Autodesk Inventor part; units mm, degrees
ref_plane "YZ Plane" through (0, 0, 0) normal (1, 0, 0) x (0, 1, 0)
ref_plane "XZ Plane" through (0, 0, 0) normal (0, 1, 0) x (-1, 0, 0)
ref_plane "XY Plane" through (0, 0, 0) normal (0, 0, 1) x (1, 0, 0)
sketch "Эскиз1" plane through (0, 0, 0) normal (0, 0, 1) x (1, 0, 0)
  line L0 (0, 0) -> (0, 7.5)
  line L1 (0, 7.5) -> (3, 7.5)
  line L2 (3, 7.5) -> (3, 2.5)
  line L3 (3, 2.5) -> (53, 2.5)
  line L4 (53, 2.5) -> (73.5263, 8)
  line L5 (128.4, 8) -> (128.4, 0)
  line L6 (128.4, 0) -> (0, 0)
  line L7 (107.9, 8) -> (107.9, 19)
  line L8 (107.9, 19) -> (106.9, 19)
  line L9 (106.9, 19) -> (106.9, 8)
  line L10 (73.5263, 8) -> (106.9, 8)
  line L11 (107.9, 8) -> (128.4, 8)
  dimension "d0" = 5
  dimension "d1" = 15
  dimension "d2" = 3
  dimension "d3" = 128.4
  dimension "d4" = 15
  dimension "d6" = 50
  dimension "d12" = 1
  dimension "d13" = 16
  dimension "d14" = 21.5
  dimension "d15" = 38
revolve "Вращение1" add sketch "Эскиз1" angle 360 about axis through (128.4, 0, 0) along (-1, 0, 0)
sketch "Эскиз2" plane through (0, 0, 0) normal (0, 1, 0) x (-1, 0, 0)
  circle A0 centre (-120.4, 0) radius 3
  line L0 (-128.4, 8) -> (-128.4, -8)
  point P0 (0, 0)
  point P1 (-128.4, 0)
  dimension "d8" = 6
  dimension "d9" = 8
extrude "Выдавливание1" cut sketch "Эскиз2" along normal through all both and the other way through all
properties part number "JF_0837B_Linear solenoid Pull 15N 12v1A Planger" material "Сталь, нержавеющая, аустенитная"
Verification items for the finished model (mm, model axes). A direction names the side the tool comes from. Give positions to 0.01 mm unless a question says otherwise; leave off trailing zeros. Loops run counter-clockwise (first coordinate to the right, second up) from the corner with the lowest first, then second, coordinate; pieces in that order, holes last.
1) Sectioned sample at C-C, the plane x = 112.5. Enter the section's corners in (y, z).
2) Depth check by flat-ended pin: pin 1 Ø10 at (x, z) = (82, 9) entering from +Y; pin 2 Ø1 at (y, z) = (-14.5, -11.5) entering from +X; pin 3 Ø10 at (y, z) = (15, 8.5) entering from -X; pin 4 Ø3.5 at (x, z) = (120.4, 0) entering from -Y. Enter the tip coordinate at first touch or a pass-through.
3) Thickness scan on line 1 along X through (y, z) = (0, 0); line 2 along Z through (x, y) = (120.4, 0); line 3 along X through (y, z) = (13, -7). Record the ranges inside material, lowest first.
4) Sectioned sample at A-A, the plane z = 0. Enter the section's corners in (x, y), then the cut area to 3 significant figures.
5) Sectioned sample at B-B, the plane y = 0. Enter the section's corners in (x, z).
6) Set-up check for faces 1 (the flat face through (107.9, -0.3, 8.2)), 2 (the cylindrical face through (122.8, 0.1, -1.8)), 3 (the flat face through (3, -2, -2)), 4 (the flat face through (0, 0, 0)), 5 (the cylindrical face through (90.45, -1.73, -7.81)): record each of +Z, -Z, +X, -X, +Y, -Y from which the full face is reachable in a straight line by a thin tool's end or side.
7) Sectioned sample at D-D, the plane y = 5.5. Count the separate pieces of the cut face and the enclosed holes in it, then the cut area to 3 significant figures.
8) Draft check along X on faces 6 (the flat face through (128.4, 0, 0)), 7 (the flat face through (106.9, -0.3, 8.2)), 8 (the cylindrical face through (107.393, 8.767, 16.856)), 9 (the conical face through (61.13, -0.61, 4.64)). Enter one of: pulls with the +X half, pulls with the -X half, needs draft (parallel to the pull), parting line crosses it, or undercut.
Answers:
1. outline: circle Ø16 at (0, 0)
2. pin 1: stops at y = 6.93
2. pin 2: stops at x = 107.9
2. pin 3: stops at x = 106.9
2. pin 4: passes through
3. line 1: x = 0 to 117.4, 123.4 to 128.4
3. line 2: z = -8 to -3, 3 to 8
3. line 3: x = 106.9 to 107.9
4. outline: (0, -7.5) - (3, -7.5) - (3, -2.5) - (53, -2.5) - (73.53, -8) - (106.9, -8) - (106.9, -19) - (107.9, -19) - (107.9, -8) - (117.4, -8) - (117.4, 8) - (107.9, 8) - (107.9, 19) - (106.9, 19) - (106.9, 8) - (73.53, 8) - (53, 2.5) - (3, 2.5) - (3, 7.5) - (0, 7.5) - close; (123.4, -8) - (128.4, -8) - (128.4, 8) - (123.4, 8) - close
4. area: 1,310 mm2
5. outline: (0, -7.5) - (3, -7.5) - (3, -2.5) - (53, -2.5) - (73.53, -8) - (106.9, -8) - (106.9, -19) - (107.9, -19) - (107.9, -8) - (128.4, -8) - (128.4, 8) - (107.9, 8) - (107.9, 19) - (106.9, 19) - (106.9, 8) - (73.53, 8) - (53, 2.5) - (3, 2.5) - (3, 7.5) - (0, 7.5) - close; hole circle Ø6 at (120.4, 0)
6. face 1: +X
6. face 2: +Y, -Y
6. face 3: none
6. face 4: +Z, -Z, -X, +Y, -Y
6. face 5: -X
7. separate pieces: 2
7. enclosed holes: 1
7. area: 734 mm2
8. face 6: pulls with the +X half
8. face 7: pulls with the -X half
8. face 8: needs draft
8. face 9: undercut
